```python
from build123d import *

# Parameters (mm, degrees)
F0_W     = 76.2
F0_H     = 76.2
F0_R     = 2.8067
F0_R_2   = 4.7625
F1_DEPTH = 6.35
F2_R     = 2.0828
F3_DEPTH = 76.201


with BuildPart() as f1:
    # F0 (on Front) → F1 (new body)
    with BuildSketch(Plane.XZ):
        Rectangle(F0_W, F0_H)
        with Locations((-12.12215, -20.99618)):
            Circle(F0_R, mode=Mode.SUBTRACT)
        with Locations((12.12215, -20.99618)):
            Circle(F0_R, mode=Mode.SUBTRACT)
        with Locations((-24.2443, 0)):
            Circle(F0_R, mode=Mode.SUBTRACT)
        with Locations((-12.12215, 20.99618)):
            Circle(F0_R, mode=Mode.SUBTRACT)
        Circle(F0_R_2, mode=Mode.SUBTRACT)
        with Locations((24.2443, 0)):
            Circle(F0_R, mode=Mode.SUBTRACT)
        with Locations((12.12215, 20.99618)):
            Circle(F0_R, mode=Mode.SUBTRACT)
    extrude(amount=F1_DEPTH)

    # F2 (on face) → F3 (cut, through all)
    with BuildSketch(Plane.XY.offset(38.1)):
        with Locations((0, -3.175)):
            Circle(F2_R)
    extrude(amount=-F3_DEPTH, mode=Mode.SUBTRACT)


solid = f1.part
```
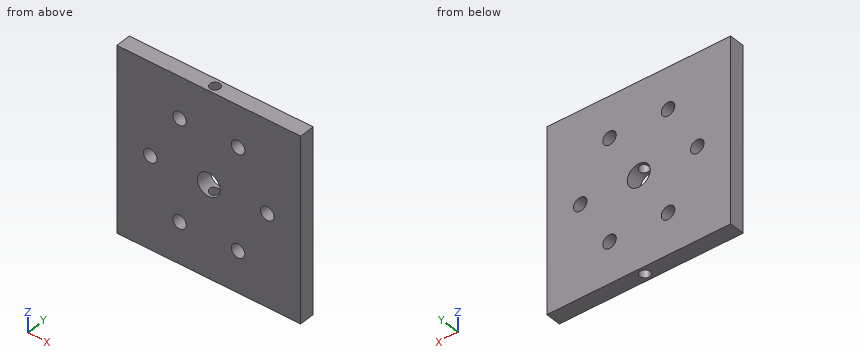
Input: part model. Units: mm. Frame: model coordinates. Coordinates: 2 decimals unless noted, no trailing zeros. Write each loop counter-clockwise with the first axis right and the second up, starting at its lowest first coordinate (ties: lowest second). Pieces come first, ordered by that corner, then holes. Notation, with made-up numbers: (21, 58.25) -> (57, 58.25) arc R18 cw to (57, 67.25) -> close; hole circle Ø4 at (26, -10.5). An arc over 180 degrees is marked (long way). Answer as a JSON object with one key per item and string values.
1. Section A-A on x = 0. Return the cut outline in (y, z).
Result set:
{"outline": "(-6.35, -38.1) -> (-5.26, -38.1) -> (-5.26, -4.76) -> (-6.35, -4.76) -> close; (-6.35, 4.76) -> (-5.26, 4.76) -> (-5.26, 38.1) -> (-6.35, 38.1) -> close; (-1.09, -38.1) -> (0, -38.1) -> (0, -4.76) -> (-1.09, -4.76) -> close; (-1.09, 4.76) -> (0, 4.76) -> (0, 38.1) -> (-1.09, 38.1) -> close"}
2. Section C-C on z = 32.5. Return the cut outline in (x, y) (3 decimals), then the cut area to 3 significant figures.
Result set:
{"outline": "(-38.1, -6.35) -> (38.1, -6.35) -> (38.1, 0) -> (-38.1, 0) -> close; hole circle Ø4.166 at (0, -3.175)", "area": "470 mm2"}
3. Material intervals for line 1 (X direction, y = -3.25, z = -29.5); line 2 (X direction, y = -5.5, z = -22); line 3 (Z direction, x = -11.5, y = -5.5), sorted ascending. Write a range as from..to.
Result set:
{"line 1": "x = -38.1..-2.08, 2.08..38.1", "line 2": "x = -38.1..-14.74, -9.5..9.5, 14.74..38.1", "line 3": "z = -38.1..-23.73, -18.26..18.26, 23.73..38.1"}
4. First-contact query: P1, Ø6.5, axis at x = -24.24, z = 0, coming from the +Y side. Flat tip, straight axial feed; report the tip coordinate or a pass-through.
Result set:
{"P1": "stops at y = 0"}
5. Section B-B on z = 0. Return the cut outline in (x, y), then the cut area to 3 significant figures.
Result set:
{"outline": "(-38.1, -6.35) -> (-27.05, -6.35) -> (-27.05, 0) -> (-38.1, 0) -> close; (-21.44, -6.35) -> (-4.76, -6.35) -> (-4.76, 0) -> (-21.44, 0) -> close; (4.76, -6.35) -> (21.44, -6.35) -> (21.44, 0) -> (4.76, 0) -> close; (27.05, -6.35) -> (38.1, -6.35) -> (38.1, 0) -> (27.05, 0) -> close", "area": "352 mm2"}
